Read the model definition and answer for the solid it produces. Units are mm, in the model's axes. Face numbers are marked on the shaded views. A direction names the side the tool comes from. Coordinates: 2 decimals unless noted, no trailing zeros. Write each loop counter-clockwise with the first axis right and the second up, starting at its lowest first coordinate (ties: lowest second). Pieces come first, ordered by that corner, then holes.
1) The part is cut by section B-B (y = -20). Determine the outline of the cut face in (x, z), then the cut area to 3 significant figures.
2) Find the intervals of material crossed by line 1 (Y direction, x = 8.7, z = 2); line 2 (Y direction, x = 0, z = 0.85); line 3 (Z direction, x = -9, y = 10), in increasing order.
3) The part is cut by section C-C (y = 15). Determine the outline of the cut face in (x, z).
4) The part is cut by section A-A (x = 8.7). Determine the outline of the cut face in (y, z), then the cut area to 3 significant figures.
5) The part is cut by section D-D (z = 5.75). Determine the outline of the cut face in (x, y), then the cut area to 3 significant figures.
6) Which of the six approach directions +Z, -Z, +X, -X, +Y, -Y give full straight-line access (tool end or side, diameter ignored) to the marked faces 1, 2 and 3?
7) Each of these flat-tipped pins is pushed along its axis until it touches: pin 1 Ø5 at (x, y) = (-8.7, 1.1) entering from +Z; pin 2 Ø2 at (x, z) = (4, 6) entering from -Y. Where does it stop, or does it pass through?
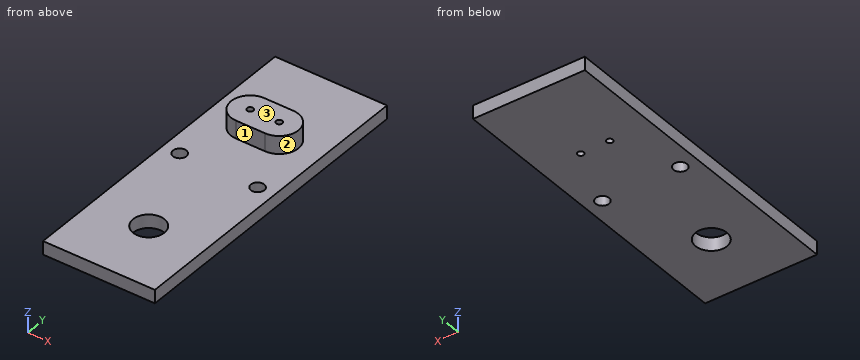
from build123d import *

# Parameters (mm, degrees)
SKETCH1_W           = 25
SKETCH1_H           = 70
SKETCH1_R           = 1.5
SKETCH1_R_2         = 3.5
BOSS_EXTRUDE1_DEPTH = 3
CUT_EXTRUDE1_REACH  = 39.286
SKETCH3_R           = 0.7
BOSS_EXTRUDE2_START = 4
SKETCH4_R           = 0.7
BOSS_EXTRUDE2_DEPTH = 4


with BuildPart() as part:
    # Sketch1 → Boss-Extrude1 (new body)
    with BuildSketch(Plane.XY):
        Rectangle(SKETCH1_W, SKETCH1_H)
        with Locations((-8.7, 1.1)):
            Circle(SKETCH1_R, mode=Mode.SUBTRACT)
        with Locations((0, -20)):
            Circle(SKETCH1_R_2, mode=Mode.SUBTRACT)
        with Locations(Location((8.7, 1.1, 0), (0, 0, 180))):
            Circle(SKETCH1_R, mode=Mode.SUBTRACT)
    extrude(amount=BOSS_EXTRUDE1_DEPTH)

    # Sketch3 → Cut-Extrude1 (cut, up to next)
    with BuildSketch(Plane.XY.offset(3), mode=Mode.PRIVATE) as cut_extrude1_sk1:
        with Locations((-3.25, 15)):
            Circle(SKETCH3_R)
    cut_extrude1_tool1 = extrude(cut_extrude1_sk1.sketch, amount=-CUT_EXTRUDE1_REACH, mode=Mode.PRIVATE) & part.part
    # Sketch3 → Cut-Extrude1 (cut, up to next)
    with BuildSketch(Plane.XY.offset(3), mode=Mode.PRIVATE) as cut_extrude1_sk2:
        with Locations((3.25, 15)):
            Circle(SKETCH3_R)
    cut_extrude1_tool2 = extrude(cut_extrude1_sk2.sketch, amount=-CUT_EXTRUDE1_REACH, mode=Mode.PRIVATE) & part.part
    add(cut_extrude1_tool1.solids().sort_by_distance((-3.25, 15, 3))[0], mode=Mode.SUBTRACT)
    add(cut_extrude1_tool2.solids().sort_by_distance((3.25, 15, 3))[0], mode=Mode.SUBTRACT)

    # Sketch4 → Boss-Extrude2 (add)
    with BuildSketch(Plane.XY.offset(3).offset(BOSS_EXTRUDE2_START)):
        with BuildLine():
            Line((-3.25, 19.269172648), (3.25, 19.269172648))
            ThreePointArc((3.25, 19.269172648), (7.519172648, 15), (3.25, 10.730827352))
            Line((3.25, 10.730827352), (-3.25, 10.730827352))
            ThreePointArc((-3.25, 10.730827352), (-7.519172648, 15), (-3.25, 19.269172648))
        make_face()
        with Locations((-3.25, 15)):
            Circle(SKETCH4_R, mode=Mode.SUBTRACT)
        with Locations((3.25, 15)):
            Circle(SKETCH4_R, mode=Mode.SUBTRACT)
    extrude(amount=-BOSS_EXTRUDE2_DEPTH)


solid = part.part
Reported:
1. outline: (-12.5, 0) - (-3.5, 0) - (-3.5, 3) - (-12.5, 3) - close; (3.5, 0) - (12.5, 0) - (12.5, 3) - (3.5, 3) - close
1. area: 54.0 mm2
2. line 1: y = -35 to -0.4, 2.6 to 35
2. line 2: y = -35 to -23.5, -16.5 to 35
2. line 3: z = 0 to 3
3. outline: (-12.5, 0) - (-3.95, 0) - (-3.95, 7) - (-7.52, 7) - (-7.52, 3) - (-12.5, 3) - close; (-2.55, 0) - (2.55, 0) - (2.55, 7) - (-2.55, 7) - close; (3.95, 0) - (12.5, 0) - (12.5, 3) - (7.52, 3) - (7.52, 7) - (3.95, 7) - close
4. outline: (-35, 0) - (-0.4, 0) - (-0.4, 3) - (-35, 3) - close; (2.6, 0) - (35, 0) - (35, 3) - (2.6, 3) - close
4. area: 201 mm2
5. outline: (-3.25, 10.73) - (3.25, 10.73) arc R4.27 ccw to (3.25, 19.27) - (-3.25, 19.27) arc R4.27 ccw to start; hole circle Ø1.4 at (-3.25, 15); hole circle Ø1.4 at (3.25, 15)
5. area: 110 mm2
6. face 1: +Z, +X, -X, -Y
6. face 2: +Z, +X
6. face 3: +Z, +X, -X, +Y, -Y
7. pin 1: stops at z = 3
7. pin 2: stops at y = 10.73
